Autodesk Inventor part; units mm, degrees
ref_plane "YZ Plane" through (0, 0, 0) normal (1, 0, 0) x (0, 1, 0)
ref_plane "XZ Plane" through (0, 0, 0) normal (0, 1, 0) x (-1, 0, 0)
ref_plane "XY Plane" through (0, 0, 0) normal (0, 0, 1) x (1, 0, 0)
sketch "Sketch1" plane through (0, 0, 0) normal (0, 1, 0) x (-1, 0, 0)
  circle A0 centre (0, 0) radius 2
  dimension "d0" = 4
extrude "Extrusion1" add sketch "Sketch1" along normal blind 1.5
sketch "Sketch2" plane through (0, 1.5, 0) normal (0, 1, 0) x (1, 0, 0)
  circle A0 centre (0, 0) radius 1.5
  dimension "d3" = 3
extrude "Extrusion2" add sketch "Sketch2" along normal blind 13
sketch "Sketch3" plane through (0, 0, 0) normal (0, -1, 0) x (1, 0, 0)
  line L0 (0.905, 0) -> (0.4525, -0.7838)
  line L1 (0.4525, -0.7838) -> (-0.4525, -0.7838)
  line L2 (-0.4525, -0.7838) -> (-0.905, 0)
  line L3 (-0.905, 0) -> (-0.4525, 0.7838)
  line L4 (-0.4525, 0.7838) -> (0.4525, 0.7838)
  line L5 (0.4525, 0.7838) -> (0.905, 0)
  point P0 (0, 0)
  point P1 (0, 0)
extrude "Extrusion3" cut sketch "Sketch3" against normal blind 1
fillet "Fillet1" radius 1 1 edges at (2, 0, 0)
thread "Thread1"
properties part number "M3x13"
Input: part model. Units: mm. Frame: model coordinates. A direction names the side the tool comes from. Round coordinates to 2 decimals unless told otherwise and drop trailing zeros. Loops run counter-clockwise (first coordinate to the right, second up) from the corner with the lowest first, then second, coordinate; pieces in that order, holes last. Notation, with made-up numbers: (31.5, 76) - (59.5, 76) arc R14 ccw to (59.5, 89) - close; hole circle Ø10 at (81.25, 86.5). An arc over 180 degrees is marked (long way). One line per item, written item: value. Start each with the question number.
(1) Draft query along X for faces 1 (the cylindrical face through (-1.5, 7.91, 0.07)), 2 (the flat face through (0, 0.5, -0.784)), 3 (the flat face through (0, 14.5, 0)). Return one class per face: +X half, -X half, draft (parallel to the pull), parting line (faces both ways), or undercut.
(2) Ray query, line 1 (Y direction, x = 0.15, z = -0.6); line 2 (X direction, y = 12.5, z = 0); line 3 (Z direction, x = 1.05, y = 4.5). Return the intervals inside material, ascending. Write a range as [from, to].
(3) Contact query for flat-ended pins moving along their axis: P1, Ø1.5, axis at x = -0.5, y = 7.5, coming from the -Z side; P2, Ø1.3, axis at x = 0.5, z = 0, coming from the -Y side; P3, Ø2, axis at y = 9, z = -1, coming from the -X side; P4, Ø1, axis at x = -1.5, y = 7.5, coming from the +Z side. Output: stop coordinate, or through.
(4) Access query for faces 4 (the flat face through (0, 1, 0)), 5 (the cylindrical face through (0.434, 1.246, 1.952)). Directions: +Z, -Z, +X, -X, +Y, -Y. A direction counts if a zero-diameter tool reaches every point of the face in a straight line with its end or side. Return the directions, or none.
(5) Section A-A, the plane y = 12.25. Return loops of the section in (x, z), plus the area to 3 significant figures.
Results below:
1. face 1: parting line
1. face 2: undercut
1. face 3: draft
2. line 1: [1, 14.5]
2. line 2: [-1.5, 1.5]
2. line 3: [-1.07, 1.07]
3. P1: z = -1.5
3. P2: y = 0
3. P3: x = -1.5
3. P4: z = 1.12
4. face 4: -Y
4. face 5: +Y, -Y
5. outline: circle Ø3 at (0, 0)
5. area: 7.07 mm^2
